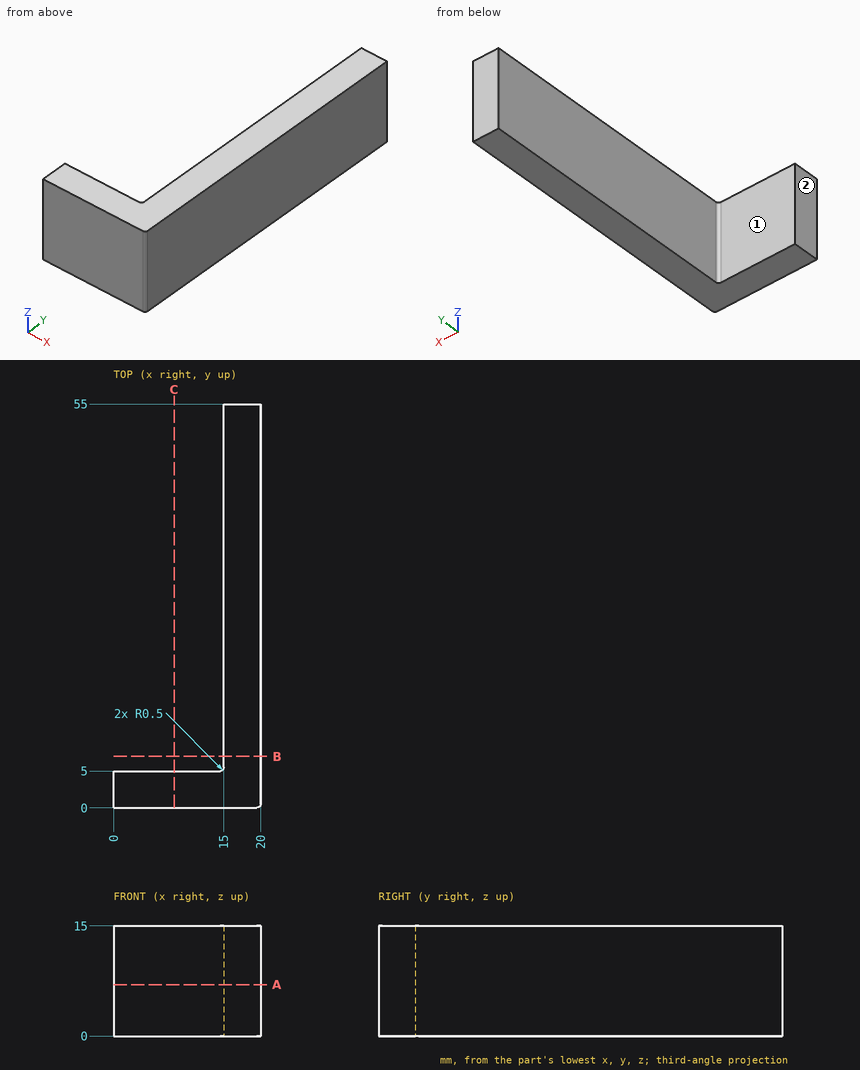
Verification items for this drawing (mm, ordinates from the low corner). A direction names the side the tool comes from. Coordinates: 2 decimals unless noted, no trailing zeros. Loops run counter-clockwise (first coordinate to the right, second up) from the corner with the lowest first, then second, coordinate; pieces in that order, holes last. Notation, with made-up numbers: (73.25, 5) -> (78.25, 5) arc R21 cw to (78.25, 43) -> close; hole circle Ø9 at (82.25, 51). An arc over 180 degrees is marked (long way). Put each result on its own line as item: value.
1. Gauge pin test, flat ends, axial feed: P1, Ø1.5, axis at y = 41, z = 11.5, coming from the -X side; P2, Ø8, axis at x = 14.5, z = 8.5, coming from the +Y side. Record the tip position at first contact, or that the pin passes through.
Result set:
P1: stops at x = 15
P2: stops at y = 55
2. Section check A-A, the plane z = 7. Record the boundary of the cut face in (x, y).
Result set:
outline: (0, 0) -> (19.5, 0) arc R0.5 ccw to (20, 0.5) -> (20, 55) -> (15, 55) -> (15, 5.5) arc R0.5 cw to (14.5, 5) -> (0, 5) -> close
3. Section check B-B, the plane y = 7. Record the boundary of the cut face in (x, z), then the cut area to 3 significant figures.
Result set:
outline: (15, 0) -> (20, 0) -> (20, 15) -> (15, 15) -> close
area: 75.0 mm^2
4. Tool access check on the marked faces 1 and 2. Record the directions out of +Z, -Z, +X, -X, +Y, -Y that give a thin tool (end or side, any length) a straight path to the whole face; none if there is none.
Result set:
face 1: +Z, -Z, -X, +Y
face 2: +Z, -Z, -X, +Y, -Y
5. Section check C-C, the plane x = 8.25. Record the boundary of the cut face in (y, z), then the cut area to 3 significant figures.
Result set:
outline: (0, 0) -> (5, 0) -> (5, 15) -> (0, 15) -> close
area: 75.0 mm^2
6. Thickness scan on line 1 (Y direction, x = 1, z = 2); line 2 (X direction, y = 44, z = 13); line 3 (Y direction, x = 14.75, z = 2.5). Record the ranges inside material, lowest first.
Result set:
line 1: y = 0 to 5
line 2: x = 15 to 20
line 3: y = 0 to 5.07
